from build123d import *

# Parameters (mm, degrees)
SKETCH_1_W                         = 4
SKETCH_1_H                         = 3.5
SM_BASE_FLANGE_1_DEPTH             = 0.4
SM_EDGE_FLANGE_1_STRIP_W           = 2.2
SM_EDGE_FLANGE_1_STRIP_H           = 0.4
SM_EDGE_FLANGE_1_STRIP_CUT_DEPTH   = 4
SM_EDGE_FLANGE_1_STRIP_2_W         = 2.2
SM_EDGE_FLANGE_1_STRIP_2_H         = 0.4
SM_EDGE_FLANGE_1_STRIP_CUT_2_DEPTH = 4
SM_EDGE_FLANGE_1_DEPTH             = 4
SM_EDGE_FLANGE_1_BEND_DEPTH        = 4
SM_EDGE_FLANGE_2_STRIP_CUT_DEPTH   = 4
SM_EDGE_FLANGE_2_STRIP_CUT_2_DEPTH = 4
SM_EDGE_FLANGE_2_DEPTH             = 4
SM_EDGE_FLANGE_2_BEND_DEPTH        = 4
SM_START                           = -2
SM_EDGE_FLANGE_3_DEPTH             = 4
SM_EDGE_FLANGE_3_2_DEPTH           = 4
SM_EDGE_FLANGE_4_STRIP_CUT_DEPTH   = 4
SM_EDGE_FLANGE_4_STRIP_CUT_2_DEPTH = 4
SM_EDGE_FLANGE_4_DEPTH             = 4
SM_EDGE_FLANGE_4_BEND_DEPTH        = 4
SM_EDGE_FLANGE_5_DEPTH             = 2.9
SM_EDGE_FLANGE_5_BEND_DEPTH        = 2.9
CUT_EXTRUDE_1_DEPTH                = 10
CUT_EXTRUDE_1_DEPTH_BACK           = 10
SKETCH_36_W                        = 1.707463823
SKETCH_36_H                        = 4.810050527
SKETCH_36_W_2                      = 1.878862713
FILLET_1_R                         = 0.55


# Read off the part's stored shape, not the designer's step: Ребро-кромка3
# Sheet-metal steps are written as plain solids
with BuildPart() as part:
    # Sketch 1 → Базовая кромка1 (new body)
    with BuildSketch(Plane(origin=(0, 0, 0), x_dir=(1, 0, 0), z_dir=(0, 1, 0))):
        Rectangle(SKETCH_1_W, SKETCH_1_H)
    extrude(amount=-SM_BASE_FLANGE_1_DEPTH)

    # Ребро-кромка1 strip (across the edge) → Ребро-кромка1 strip cut (cut)
    with BuildSketch(Plane(origin=(-2, 0, 1.75), x_dir=(0, 0, -1), z_dir=(1, 0, 0))):
        with Locations((-0.8, -0.2)):
            Rectangle(SM_EDGE_FLANGE_1_STRIP_W, SM_EDGE_FLANGE_1_STRIP_H)
    extrude(amount=SM_EDGE_FLANGE_1_STRIP_CUT_DEPTH, mode=Mode.SUBTRACT)

    # Ребро-кромка1 strip 2 (across the edge) → Ребро-кромка1 strip cut 2 (cut)
    with BuildSketch(Plane(origin=(2, 0, -1.75), x_dir=(0, 0, 1), z_dir=(-1, 0, 0))):
        with Locations((-0.8, -0.2)):
            Rectangle(SM_EDGE_FLANGE_1_STRIP_2_W, SM_EDGE_FLANGE_1_STRIP_2_H)
    extrude(amount=SM_EDGE_FLANGE_1_STRIP_CUT_2_DEPTH, mode=Mode.SUBTRACT)

    # Ребро-кромка1 section (across the edge) → Ребро-кромка1 (add)
    with BuildSketch(Plane(origin=(-2, 0, 1.75), x_dir=(0, 0, -1), z_dir=(1, 0, 0))):
        with BuildLine():
            Line((-0.4, 0.3), (-0.4, 2.5))
            Line((-0.4, 2.5), (0, 2.5))
            Line((0, 2.5), (0, 0.3))
            ThreePointArc((0, 0.3), (0.087867966, 0.087867966), (0.3, 0))
            Line((0.3, 0), (0.3, -0.4))
            ThreePointArc((0.3, -0.4), (-0.194974747, -0.194974747), (-0.4, 0.3))
        make_face()
    extrude(amount=SM_EDGE_FLANGE_1_DEPTH)

    # Ребро-кромка1 section 2 (across the edge) → Ребро-кромка1 bend (add)
    with BuildSketch(Plane(origin=(2, 0, -1.75), x_dir=(0, 0, 1), z_dir=(-1, 0, 0))):
        with BuildLine():
            Line((-0.4, 0.3), (-0.4, 2.5))
            Line((-0.4, 2.5), (0, 2.5))
            Line((0, 2.5), (0, 0.3))
            ThreePointArc((0, 0.3), (0.087867966, 0.087867966), (0.3, 0))
            Line((0.3, 0), (0.3, -0.4))
            ThreePointArc((0.3, -0.4), (-0.194974747, -0.194974747), (-0.4, 0.3))
        make_face()
    extrude(amount=SM_EDGE_FLANGE_1_BEND_DEPTH)

    # Ребро-кромка2 strip (across the edge) → Ребро-кромка2 strip cut (cut)
    with BuildSketch(Plane(origin=(2, 2.5, 2.15), x_dir=(0, -0.49999999999999795, 0.8660254037844398), z_dir=(-1, 0, 0))):
        Polygon((-2.878460969, 4.185640646), (-0.078460969, -0.664101615), (0.267949192, -0.464101615), (-2.532050808, 4.385640646), align=None)
    extrude(amount=SM_EDGE_FLANGE_2_STRIP_CUT_DEPTH, mode=Mode.SUBTRACT)

    # Ребро-кромка2 strip 2 (across the edge) → Ребро-кромка2 strip cut 2 (cut)
    with BuildSketch(Plane(origin=(-2, 2.5, -2.15), x_dir=(0, -0.49999999999999495, -0.8660254037844416), z_dir=(1, 0, 0))):
        Polygon((-2.878460969, 4.185640646), (-0.078460969, -0.664101615), (0.267949192, -0.464101615), (-2.532050808, 4.385640646), align=None)
    extrude(amount=SM_EDGE_FLANGE_2_STRIP_CUT_2_DEPTH, mode=Mode.SUBTRACT)

    # Ребро-кромка2 section (across the edge) → Ребро-кромка2 (add)
    with BuildSketch(Plane(origin=(2, 2.5, 2.15), x_dir=(0, -0.49999999999999795, 0.8660254037844398), z_dir=(-1, 0, 0))):
        with BuildLine():
            Line((-0.4, 0.535898385), (-0.4, 2))
            Line((-0.4, 2), (0, 2))
            Line((0, 2), (0, 0.535898385))
            ThreePointArc((0, 0.535898385), (0.068148347, 0.018260295), (0.267949192, -0.464101615))
            Line((0.267949192, -0.464101615), (-0.078460969, -0.664101615))
            ThreePointArc((-0.078460969, -0.664101615), (-0.318221983, -0.085267323), (-0.4, 0.535898385))
        make_face()
    extrude(amount=SM_EDGE_FLANGE_2_DEPTH)

    # Ребро-кромка2 section 2 (across the edge) → Ребро-кромка2 bend (add)
    with BuildSketch(Plane(origin=(-2, 2.5, -2.15), x_dir=(0, -0.49999999999999495, -0.8660254037844416), z_dir=(1, 0, 0))):
        with BuildLine():
            Line((-0.4, 0.535898385), (-0.4, 2))
            Line((-0.4, 2), (0, 2))
            Line((0, 2), (0, 0.535898385))
            ThreePointArc((0, 0.535898385), (0.068148347, 0.018260295), (0.267949192, -0.464101615))
            Line((0.267949192, -0.464101615), (-0.078460969, -0.664101615))
            ThreePointArc((-0.078460969, -0.664101615), (-0.318221983, -0.085267323), (-0.4, 0.535898385))
        make_face()
    extrude(amount=SM_EDGE_FLANGE_2_BEND_DEPTH)

    # Ребро-кромка3 outline → Ребро-кромка3 (cut)
    with BuildSketch(Plane.YZ.offset(SM_START)):
        with BuildLine():
            ThreePointArc((3.232050808, 2.572649731), (3.785814556, 2.80554739), (4.380068552, 2.893625747))
            Line((4.380068552, 2.893625747), (4.232050808, 3.15))
            Line((4.232050808, 3.15), (3.232050808, 2.572649731))
        make_face()
        with BuildLine():
            Line((4.232050808, -3.15), (4.380068552, -2.893625747))
            ThreePointArc((4.380068552, -2.893625747), (3.785814556, -2.80554739), (3.232050808, -2.572649731))
            Line((3.232050808, -2.572649731), (4.232050808, -3.15))
        make_face()
    extrude(amount=SM_EDGE_FLANGE_3_DEPTH, mode=Mode.SUBTRACT)

    # Sm Edge Flange 3 2 outline → Sm Edge Flange 3 2 (add)
    with BuildSketch(Plane.YZ.offset(SM_START)):
        with BuildLine():
            Line((6.364101615, 2.15), (5.632050808, 2.572649731))
            ThreePointArc((5.632050808, 2.572649731), (5.028073111, 2.819002177), (4.380068552, 2.893625747))
            Line((4.380068552, 2.893625747), (4.432050808, 2.803589838))
            Line((4.432050808, 2.803589838), (3.432050808, 2.226239569))
            ThreePointArc((3.432050808, 2.226239569), (4.432050808, 2.494188762), (5.432050808, 2.226239569))
            Line((5.432050808, 2.226239569), (6.164101615, 1.803589838))
            Line((6.164101615, 1.803589838), (6.364101615, 2.15))
        make_face()
        with BuildLine():
            ThreePointArc((4.380068552, -2.893625747), (5.028073111, -2.819002177), (5.632050808, -2.572649731))
            Line((5.632050808, -2.572649731), (6.364101615, -2.15))
            Line((6.364101615, -2.15), (6.164101615, -1.803589838))
            Line((6.164101615, -1.803589838), (5.432050808, -2.226239569))
            ThreePointArc((5.432050808, -2.226239569), (4.432050808, -2.494188762), (3.432050808, -2.226239569))
            Line((3.432050808, -2.226239569), (4.432050808, -2.803589838))
            Line((4.432050808, -2.803589838), (4.380068552, -2.893625747))
        make_face()
    extrude(amount=SM_EDGE_FLANGE_3_2_DEPTH)

    # Ребро-кромка4 strip (across the edge) → Ребро-кромка4 strip cut (cut)
    with BuildSketch(Plane(origin=(2, 6.364101615, 2.15), x_dir=(0, -0.4999999999999979, 0.8660254037844399), z_dir=(-1, 0, 0))):
        Polygon((-1.955255888, 0.666987298), (-0.05, -0.433012702), (0.15, -0.08660254), (-1.755255888, 1.01339746), align=None)
    extrude(amount=SM_EDGE_FLANGE_4_STRIP_CUT_DEPTH, mode=Mode.SUBTRACT)

    # Ребро-кромка4 strip 2 (across the edge) → Ребро-кромка4 strip cut 2 (cut)
    with BuildSketch(Plane(origin=(-2, 6.364101615, -2.15), x_dir=(0, -0.4999999999999948, -0.8660254037844417), z_dir=(1, 0, 0))):
        Polygon((-1.955255888, 0.666987298), (-0.05, -0.433012702), (0.15, -0.08660254), (-1.755255888, 1.01339746), align=None)
    extrude(amount=SM_EDGE_FLANGE_4_STRIP_CUT_2_DEPTH, mode=Mode.SUBTRACT)

    # Ребро-кромка4 section (across the edge) → Ребро-кромка4 (add)
    with BuildSketch(Plane(origin=(2, 6.364101615, 2.15), x_dir=(0, -0.4999999999999979, 0.8660254037844399), z_dir=(-1, 0, 0))):
        with BuildLine():
            Line((-0.4, 0.173205081), (-0.4, 1.5))
            Line((-0.4, 1.5), (0, 1.5))
            Line((0, 1.5), (0, 0.173205081))
            ThreePointArc((0, 0.173205081), (0.040192379, 0.023205081), (0.15, -0.08660254))
            Line((0.15, -0.08660254), (-0.05, -0.433012702))
            ThreePointArc((-0.05, -0.433012702), (-0.306217783, -0.176794919), (-0.4, 0.173205081))
        make_face()
    extrude(amount=SM_EDGE_FLANGE_4_DEPTH)

    # Ребро-кромка4 section 2 (across the edge) → Ребро-кромка4 bend (add)
    with BuildSketch(Plane(origin=(-2, 6.364101615, -2.15), x_dir=(0, -0.4999999999999948, -0.8660254037844417), z_dir=(1, 0, 0))):
        with BuildLine():
            Line((-0.4, 0.173205081), (-0.4, 1.5))
            Line((-0.4, 1.5), (0, 1.5))
            Line((0, 1.5), (0, 0.173205081))
            ThreePointArc((0, 0.173205081), (0.040192379, 0.023205081), (0.15, -0.08660254))
            Line((0.15, -0.08660254), (-0.05, -0.433012702))
            ThreePointArc((-0.05, -0.433012702), (-0.306217783, -0.176794919), (-0.4, 0.173205081))
        make_face()
    extrude(amount=SM_EDGE_FLANGE_4_BEND_DEPTH)

    # Ребро-кромка5 section (across the edge) → Ребро-кромка5 (add)
    with BuildSketch(Plane(origin=(2.4, -0.4, -1.45), x_dir=(-1, 0, 0), z_dir=(0, 0, 1))):
        with BuildLine():
            Line((-0.4, 0.4), (-0.4, 5.8))
            Line((-0.4, 5.8), (0, 5.8))
            Line((0, 5.8), (0, 0.4))
            ThreePointArc((0, 0.4), (0.117157288, 0.117157288), (0.4, 0))
            Line((0.4, 0), (0.4, -0.4))
            ThreePointArc((0.4, -0.4), (-0.165685425, -0.165685425), (-0.4, 0.4))
        make_face()
    extrude(amount=SM_EDGE_FLANGE_5_DEPTH)

    # Ребро-кромка5 section 2 (across the edge) → Ребро-кромка5 bend (add)
    with BuildSketch(Plane(origin=(-2.4, -0.4, 1.45), x_dir=(1, 0, 0), z_dir=(0, 0, -1))):
        with BuildLine():
            Line((-0.4, 0.4), (-0.4, 5.8))
            Line((-0.4, 5.8), (0, 5.8))
            Line((0, 5.8), (0, 0.4))
            ThreePointArc((0, 0.4), (0.117157288, 0.117157288), (0.4, 0))
            Line((0.4, 0), (0.4, -0.4))
            ThreePointArc((0.4, -0.4), (-0.165685425, -0.165685425), (-0.4, 0.4))
        make_face()
    extrude(amount=SM_EDGE_FLANGE_5_BEND_DEPTH)

    # Эскиз36 → Вырез-Вытянуть1 (cut, two sides: drawn at the far end of the back side and taken through both)
    with BuildSketch(Plane(origin=(0, 0, 0), x_dir=(0, 0, -1), z_dir=(1, 0, 0)).offset(-CUT_EXTRUDE_1_DEPTH_BACK)):
        with Locations((1.453731912, -5.305025264)):
            Rectangle(SKETCH_36_W, SKETCH_36_H)
        with Locations((-1.539431357, -5.305025264)):
            Rectangle(SKETCH_36_W_2, SKETCH_36_H)
    extrude(amount=CUT_EXTRUDE_1_DEPTH + CUT_EXTRUDE_1_DEPTH_BACK, mode=Mode.SUBTRACT)

    # Скругление1
    fillet_1_edges = [part.edges().sort_by_distance(p)[0] for p in [
        (-2.6, -6.2, -0.6),
        (2.6, -6.2, -0.6),
        (-2.6, -6.2, 0.6),
        (2.6, -6.2, 0.6),
    ]]
    fillet(fillet_1_edges, radius=FILLET_1_R)


solid = part.part
Part model, mm, in its own coordinate system. A direction names the side the tool comes from. Give positions to 0.01 mm unless a question says otherwise; leave off trailing zeros. Loops run counter-clockwise (first coordinate to the right, second up) from the corner with the lowest first, then second, coordinate; pieces in that order, holes last.
(1) Pull direction Z, two halves, no side cores. Call faces 6 (the cylindrical face through (0.03, 2.49, 2.22)), 7 (the flat face through (0, 0, 0)), 8 (the flat face through (0, -0.4, 0)): pulls with the +Z half, pulls with the -Z half, needs draft (parallel to the pull), parting line crosses it, or undercut.
Return value:
face 6: pulls with the +Z half
face 7: undercut
face 8: needs draft
(2) 3-axis set-ups, long thin cutter, end or side, ignore diameter. For faces 1 (the flat face through (0, 1, -1.75)), 2 (the cylindrical face through (-0.03, 2.58, -1.83)), 3 (the flat face through (0, 1, 2.15)), 4 (the flat face through (-2.6, -1.5, -1.45)), 5 (the flat face through (2.6, -1.5, 1.45)): which of +Z, -Z, +X, -X, +Y, -Y reach the whole face in a straight line?
Return value:
face 1: +X, -X, +Y
face 2: +X, -X
face 3: +Z, +X, -X, -Y
face 4: -Z, -X, +Y, -Y
face 5: +Z, +X, +Y, -Y
(3) Pin check, flat tips, straight feed: pin 1 (0.8 mm diameter, centred on x = -0.5, y = 1, fed in from -Z); pin 2 (2.5 mm diameter, centred on x = -1, z = 0, fed in from -Y); pin 3 (1.6 mm diameter, centred on y = 4, z = 2, fed in from +X). Stop position of each tip, or through.
Return value:
pin 1: stops at z = -2.15
pin 2: stops at y = -0.49
pin 3: stops at x = 2
(4) Band-saw the part on C-C (y = 0.75). Write the cut outline in (x, z).
Return value:
outline: (-2, -2.15) - (2, -2.15) - (2, -1.75) - (-2, -1.75) - close; (-2, 1.75) - (2, 1.75) - (2, 2.15) - (-2, 2.15) - close
(5) Drill centre lines: line 1 along Z through (x, y) = (-1.8, 0.5); line 2 along X through (y, z) = (-2, -0.3); line 3 along Z through (x, y) = (1.05, 2.5). Where is each one in solid material? Low to high.
Return value:
line 1: z = -2.15 to -1.75, 1.75 to 2.15
line 2: x = -2.8 to -2.4, 2.4 to 2.8
line 3: z = -2.22 to -1.81, 1.81 to 2.22
(6) Band-saw the part on B-B (z = 1.15). Write the cut outline in (x, y), and give its area (3 significant figures).
Return value:
outline: (-2.8, -2.9) - (-2.4, -2.9) - (-2.4, -0.8) arc R0.4 cw to (-2, -0.4) - (2, -0.4) arc R0.4 cw to (2.4, -0.8) - (2.4, -2.9) - (2.8, -2.9) - (2.8, -0.8) arc R0.8 ccw to (2, 0) - (-2, 0) arc R0.8 ccw to (-2.8, -0.8) - close
area: 4.03 mm2
(7) Band-saw the part on A-A (y = -2.75). Write the cut outline in (x, z).
Return value:
outline: (-2.8, -1.45) - (-2.4, -1.45) - (-2.4, 1.45) - (-2.8, 1.45) - close; (2.4, -1.45) - (2.8, -1.45) - (2.8, 1.45) - (2.4, 1.45) - close
